Can you work these out from the model? Positions are in its coordinate system, mm. A direction names the side the tool comes from. Give positions to 0.01 mm unless a question says otherwise; leave off trailing zeros. Order: outer loops, then holes, each group sorted by start corner. A loop starts at its lowest first (then second) coordinate and runs counter-clockwise, first axis right, second up. Notation, with made-up numbers: (38, 33.25) - (74, 33.25) arc R27 ccw to (74, 72.25) - close; hole circle Ø10 at (-23, -38.75). An arc over 180 degrees is marked (long way). Return JSON: item names as keys, results as strings.
```python
from build123d import *

# Parameters (mm, degrees)
SKETCH_2_R          = 20
SKETCH_5_R          = 50
EXTRUDE_1_DEPTH     = 3
SKETCH_6_R          = 15
SKETCH_6_R_2        = 9.261363372
CUT_EXTRUDE_1_DEPTH = 3
SKETCH_8_R          = 50
EXTRUDE_2_DEPTH     = 3
SKETCH_9_R          = 15
SKETCH_9_R_2        = 6.547134089
CUT_EXTRUDE_2_DEPTH = 3


with BuildPart() as part:
    # 扫描1: sweep along a path in 草图1
    with BuildLine(Plane.XY) as sweep_1_path:
        ThreePointArc((-42.426406871, 42.426406871), (-55.432771951, 22.961005942), (-60, 0))
    # 草图2 → 扫描1 (sweep)
    with BuildSketch(Plane(origin=(0, 0, 0), x_dir=(1, 0, 0), z_dir=(0, 1, 0))):
        with Locations((-60, 0)):
            Circle(SKETCH_2_R)
    sweep(path=sweep_1_path.line)

    # 草图5 → 凸台-拉伸1 (add)
    with BuildSketch(Plane(origin=(0, 0, 0), x_dir=(0, 0, -1), z_dir=(0.7071067811865434, 0.7071067811865517, 0))):
        with Locations(Location((0, 60, 0), (0, 0, 90))):
            Circle(SKETCH_5_R)
    extrude(amount=EXTRUDE_1_DEPTH)

    # 草图6 → 切除-拉伸1 (cut)
    with BuildSketch(Plane(origin=(2.121320344, 2.121320344, 0), x_dir=(0, 0, -1), z_dir=(0.7071067811865434, 0.7071067811865517, 0))):
        with Locations(Location((0, 60, 0), (0, 0, 90))):
            Circle(SKETCH_6_R)
        with Locations(Location((0, 97.5, 0), (0, 0, 90))):
            Circle(SKETCH_6_R_2)
        with Locations(Location((37.5, 60, 0), (0, 0, 90))):
            Circle(SKETCH_6_R_2)
        with Locations(Location((0, 22.5, 0), (0, 0, 90))):
            Circle(SKETCH_6_R_2)
        with Locations(Location((-37.5, 60, 0), (0, 0, 90))):
            Circle(SKETCH_6_R_2)
    extrude(amount=-CUT_EXTRUDE_1_DEPTH, mode=Mode.SUBTRACT)

    # 草图8 → 凸台-拉伸2 (add)
    with BuildSketch(Plane.XZ):
        with Locations(Location((-60, 0, 0), (0, 0, 270))):
            Circle(SKETCH_8_R)
    extrude(amount=EXTRUDE_2_DEPTH)

    # 草图9 → 切除-拉伸2 (cut)
    with BuildSketch(Plane.XZ.offset(3)):
        with Locations(Location((-60, 0, 0), (0, 0, 270))):
            Circle(SKETCH_9_R)
        with Locations(Location((-60, 37.5, 0), (0, 0, 270))):
            Circle(SKETCH_9_R_2)
        with Locations(Location((-22.5, 0, 0), (0, 0, 270))):
            Circle(SKETCH_9_R_2)
        with Locations(Location((-60, -37.5, 0), (0, 0, 270))):
            Circle(SKETCH_9_R_2)
        with Locations(Location((-97.5, 0, 0), (0, 0, 270))):
            Circle(SKETCH_9_R_2)
    extrude(amount=-CUT_EXTRUDE_2_DEPTH, mode=Mode.SUBTRACT)


solid = part.part
```
1. Thinking about a two-plate mould opening in Z: for faces 4 (the face through (-108.81, -1.48, 10.84)), 5 (the face through (-48, -3, -10)), 6 (the face through (-40.498, 42.649, 46.683)), which applies, +Z half, -Z half, draft (parallel to the pull), parting line (faces both ways), or undercut?
Checks:
{"face 4": "parting line", "face 5": "draft", "face 6": "undercut"}
2. Suppose I cut it at B-B (x = -13.5). State how many separate pieces and enclosed holes the cut face has, plus the area to 3 significant figures.
Checks:
{"separate pieces": "3", "enclosed holes": "0", "area": "295 mm^2"}
3. If I drill on L1, parallel to X at y = -2.2, z = 0; L2, parallel to Y at x = -78, z = -43; L3, parallel to X at y = -1.85, z = 37.5, over which ranges is the centre line in solid material (lowest first)? Write a range as [from, to].
Checks:
{"L1": "[-110, -104.05], [-90.95, -75], [-45, -29.05], [-15.95, -10]", "L2": "[-3, 0]", "L3": "[-93.07, -66.55], [-53.45, -26.93]"}
4. On a 3-axis mill with a long thin cutter (end or side, diameter ignored), from which of +Z, -Z, +X, -X, +Y, -Y can I reach the whole of each face in a straight line? I mean faces 1 (the face through (-47.67, 51.91, 11.81)), 2 (the face through (-53.51, -1.52, 38.35)), 3 (the face through (-82, 0, 1)). Say none if no direction works.
Checks:
{"face 1": "+Z, -Z, +X, +Y", "face 2": "-Y", "face 3": "none"}
5. Suppose I cut it at C-C (z = 18). List the corners of the cut face in (x, y) for me.
Checks:
{"outline": "(-106.65, -3) - (-13.35, -3) - (-13.35, 0) - (-51.28, 0) arc R51.28 cw to (-36.26, 36.26) - (-9.44, 9.44) - (-7.32, 11.56) - (-73.29, 77.53) - (-75.41, 75.41) - (-48.59, 48.59) arc R68.72 ccw to (-68.72, 0) - (-106.65, 0) - close"}
6. Suppose I cut it at A-A (z = 37.5). List the corners of the cut face in (x, y) for me, plus the area to 3 significant figures.
Checks:
{"outline": "(-93.07, -3) - (-66.55, -3) - (-66.55, 0) - (-93.07, 0) - close; (-65.81, 65.81) - (-48.98, 48.98) - (-46.85, 51.1) - (-63.69, 67.93) - close; (-53.45, -3) - (-26.93, -3) - (-26.93, 0) - (-53.45, 0) - close; (-35.88, 35.88) - (-19.04, 19.04) - (-16.92, 21.16) - (-33.76, 38) - close", "area": "302 mm^2"}
7. For pin 1 Ø8 at (x, z) = (-60, -37.5) entering from -Y; pin 2 Ø1 at (y, z) = (7.5, -8) entering from -X; pin 3 Ø5 at (x, y) = (-28, 30.5) entering from +Z, each with a flat end and sliding along its axis, tell me the tip position at first contact or that it passes through.
Checks:
{"pin 1": "y = 56", "pin 2": "x = -78.19", "pin 3": "z = 47.33"}
